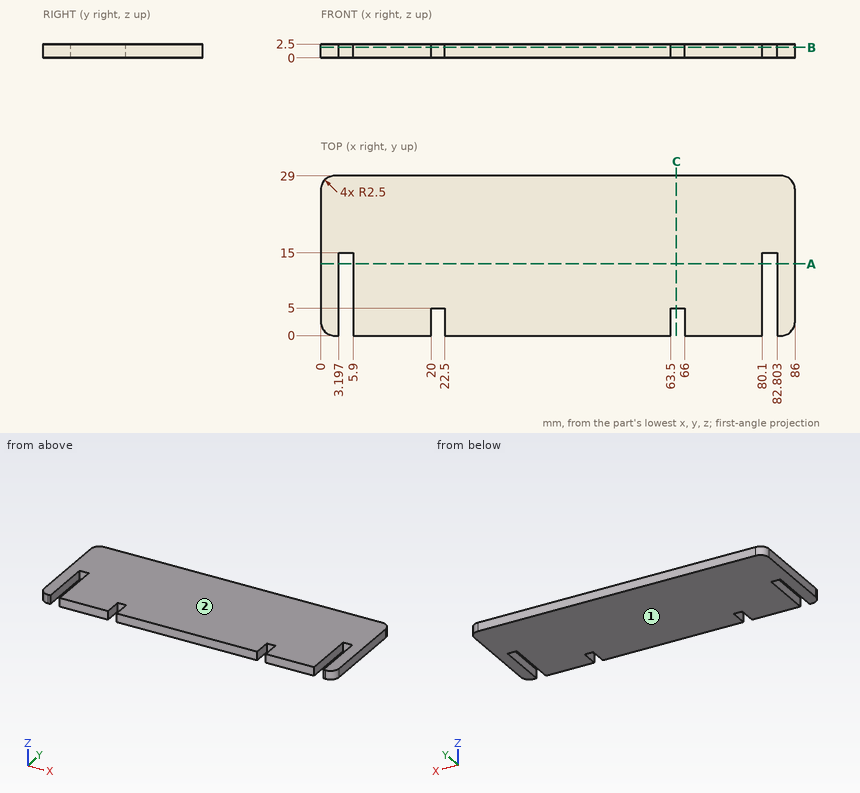
Design review of the part shown in the three views and the two pictorial views. Dimensions are in mm from the part's minimum x, y and z. Coordinates: 2 decimals unless noted, no trailing zeros. Write each loop counter-clockwise with the first axis right and the second up, starting at its lowest first coordinate (ties: lowest second). Pieces come first, ordered by that corner, then holes.
1) We need section B-B on z = 1.9. State the section outline as (x, y) points, then the cut area to 3 significant figures.
2) We need section C-C on x = 64.5. State the section outline as (y, z) points, then the cut area to 3 significant figures.
3) To check wall thickness, follow probe 1 along X at (y, z) = (3, 0.8); probe 2 along X at (y, z) = (6.75, 1.95); probe 3 along X at (y, z) = (2, 2.35). State the ranges of each line that lie inside material, in increasing order.
4) Clearance check with flat-ended pins moving along their axes: pin 1 Ø0.8 at (x, z) = (64.5, 1) entering from -Y; pin 2 Ø0.8 at (x, z) = (81.5, 1.5) entering from -Y; pin 3 Ø0.8 at (y, z) = (2, 1.5) entering from -X. State where each tip first meets the part, or that it passes through.
5) We need section A-A on y = 13. State the section outline as (x, z) points, then the cut area to 4 significant figures.
6) The part is to be moulded in two halves that separate along Z. For the marked faces 1 and 2, say which applies: pulls with the +Z half, pulls with the -Z half, needs draft (parallel to the pull), parting line crosses it, or undercut.
Answer list:
1. outline: (0, 2.5) arc R2.5 ccw to (2.5, 0) - (3.2, 0) - (3.2, 15) - (5.9, 15) - (5.9, 0) - (20, 0) - (20, 5) - (22.5, 5) - (22.5, 0) - (63.5, 0) - (63.5, 5) - (66, 5) - (66, 0) - (80.1, 0) - (80.1, 15) - (82.8, 15) - (82.8, 0) - (83.5, 0) arc R2.5 ccw to (86, 2.5) - (86, 26.5) arc R2.5 ccw to (83.5, 29) - (2.5, 29) arc R2.5 ccw to (0, 26.5) - close
1. area: 2,380 mm2
2. outline: (5, 0) - (29, 0) - (29, 2.5) - (5, 2.5) - close
2. area: 60.0 mm2
3. probe 1: x = 0 to 3.2, 5.9 to 20, 22.5 to 63.5, 66 to 80.1, 82.8 to 86
3. probe 2: x = 0 to 3.2, 5.9 to 80.1, 82.8 to 86
3. probe 3: x = 0.05 to 3.2, 5.9 to 20, 22.5 to 63.5, 66 to 80.1, 82.8 to 85.95
4. pin 1: stops at y = 5
4. pin 2: stops at y = 15
4. pin 3: stops at x = 0
5. outline: (0, 0) - (3.2, 0) - (3.2, 2.5) - (0, 2.5) - close; (5.9, 0) - (80.1, 0) - (80.1, 2.5) - (5.9, 2.5) - close; (82.8, 0) - (86, 0) - (86, 2.5) - (82.8, 2.5) - close
5. area: 201.5 mm2
6. face 1: pulls with the -Z half
6. face 2: pulls with the +Z half
